```python
from build123d import *

# Parameters (mm, degrees)
SKETCH1_W                   = 82
SKETCH1_H                   = 30
SKETCH1_R                   = 7
SKETCH1_R_2                 = 2.1
BOSS_EXTRUDE1_DEPTH         = 25.4
SKETCH2_W                   = 20
SKETCH2_H                   = 12.7
CUT_EXTRUDE1_DEPTH          = 32
FILLET1_R                   = 1
TAP_DRILL_FOR_M4X0_7_TAP1_D = 3.3


with BuildPart() as part:
    # Sketch1 → Boss-Extrude1 (new body)
    with BuildSketch(Plane(origin=(0, 0, 0), x_dir=(1, 0, 0), z_dir=(0, 1, 0))):
        with Locations((-26, 0)):
            Rectangle(SKETCH1_W, SKETCH1_H)
        with Locations(Location((0, 0, 0), (0, 0, 270))):
            Circle(SKETCH1_R, mode=Mode.SUBTRACT)
        with Locations(Location((-60, 0, 0), (0, 0, 270))):
            Circle(SKETCH1_R_2, mode=Mode.SUBTRACT)
    extrude(amount=-BOSS_EXTRUDE1_DEPTH)

    # Sketch2 → Cut-Extrude1 (cut)
    with BuildSketch(Plane(origin=(0, 0, 15), x_dir=(-1, 0, 0), z_dir=(0, 0, -1))):
        with Locations((57, -12.7)):
            Rectangle(SKETCH2_W, SKETCH2_H)
    extrude(amount=CUT_EXTRUDE1_DEPTH, mode=Mode.SUBTRACT)

    # Fillet1
    fillet1_edges = [part.edges().sort_by_distance(p)[0] for p in [
        (-67, -3.175, -15),
        (-67, -3.175, 15),
        (15, -12.7, 15),
        (-67, -22.225, 15),
        (-67, -22.225, -15),
        (15, -12.7, -15),
    ]]
    fillet(fillet1_edges, radius=FILLET1_R)

    # Tap Drill for M4x0.7 Tap1 (through all)
    with Locations(Plane(origin=(0, -12.7, 15), x_dir=(1, 0, 0), z_dir=(0, 0, 1))):
        with Locations((0, 0)):
            Hole(TAP_DRILL_FOR_M4X0_7_TAP1_D / 2)


solid = part.part
```
The model under review builds one solid part; all positions refer to its coordinate system, in mm. A direction names the side the tool comes from. Give positions to 0.01 mm unless a question says otherwise; leave off trailing zeros. Write each loop counter-clockwise with the first axis right and the second up, starting at its lowest first coordinate (ties: lowest second). Pieces come first, ordered by that corner, then holes.
(1) The part is to be moulded in two halves that separate along Y. For faces 1 (the flat face through (-67, -3, 0)), 2 (the flat face through (-57, -6.35, 0)), 3 (the flat face through (-27, 0, 0)), 4 (the flat face through (-57, -19.05, 0)), say which applies: released by +Y, released by -Y, zero draft, split by the parting line, or undercut.
(2) To check wall thickness, follow L1, parallel to X at y = -2, z = 0; L2, parallel to X at y = -12.7, z = -9.75; L3, parallel to Y at x = 0, z = -9. State the ranges of each line that lie inside material, in increasing order.
(3) For P1, Ø1, axis at y = -12.5, z = 5.5, coming from the -X side, flat-tipped, find the tip position at first contact; note if it passes through.
(4) Consider section D-D, the plane y = -12.7. Give the boundary of the cut face in (x, z), and give its area (3 significant figures).
(5) Consider section C-C, the plane y = -1.75. Give the boundary of the cut face in (x, z).
(6) Consider section B-B, the plane z = 0. Give the boundary of the cut face in (x, y), and give its area (3 significant figures).
(7) Consider section A-A, the plane x = -60. Give the boundary of the cut face in (y, z).
(8) Tool access review of faces 5 (the flat face through (-47, -13, 0)), 6 (the flat face through (-67, -22, 0)): name each direction out of +Z, -Z, +X, -X, +Y, -Y from which nothing blocks a thin tool from reaching the whole face with its end or side.
Returned:
1. face 1: zero draft
1. face 2: undercut
1. face 3: released by +Y
1. face 4: undercut
2. L1: x = -67 to -62.1, -57.9 to -7, 7 to 15
2. L2: x = -47 to -1.65, 1.65 to 15
2. L3: y = -25.4 to -14.35, -11.05 to 0
3. P1: stops at x = -47
4. outline: (-47, -15) - (-1.65, -15) - (-1.65, -6.8) arc R7 cw to (-1.65, 6.8) - (-1.65, 15) - (-47, 15) - close; (1.65, -15) - (14, -15) arc R1 ccw to (15, -14) - (15, 14) arc R1 ccw to (14, 15) - (1.65, 15) - (1.65, 6.8) arc R7 cw to (1.65, -6.8) - close
4. area: 1,650 mm2
5. outline: (-67, -14) arc R1 ccw to (-66, -15) - (14, -15) arc R1 ccw to (15, -14) - (15, 14) arc R1 ccw to (14, 15) - (-66, 15) arc R1 ccw to (-67, 14) - close; hole circle Ø4.2 at (-60, 0); hole circle Ø14 at (0, 0)
6. outline: (-67, -25.4) - (-62.1, -25.4) - (-62.1, -19.05) - (-67, -19.05) - close; (-67, -6.35) - (-62.1, -6.35) - (-62.1, 0) - (-67, 0) - close; (-57.9, -25.4) - (-7, -25.4) - (-7, 0) - (-57.9, 0) - (-57.9, -6.35) - (-47, -6.35) - (-47, -19.05) - (-57.9, -19.05) - close; (7, -25.4) - (15, -25.4) - (15, 0) - (7, 0) - close
6. area: 1,420 mm2
7. outline: (-25.4, -15) - (-19.05, -15) - (-19.05, -2.1) - (-25.4, -2.1) - close; (-25.4, 2.1) - (-19.05, 2.1) - (-19.05, 15) - (-25.4, 15) - close; (-6.35, -15) - (0, -15) - (0, -2.1) - (-6.35, -2.1) - close; (-6.35, 2.1) - (0, 2.1) - (0, 15) - (-6.35, 15) - close
8. face 5: +Z, -Z, -X
8. face 6: +Z, -Z, -X, +Y, -Y
